For this review, take the finished solid that the model builds, in its own axes (mm). A direction names the side the tool comes from. Give positions to 0.01 mm unless a question says otherwise; leave off trailing zeros. Loops run counter-clockwise (first coordinate to the right, second up) from the corner with the lowest first, then second, coordinate; pieces in that order, holes last. Notation, with made-up numbers: (-23, 48.5) - (19, 48.5) arc R17 cw to (19, 62.5) - close; hole circle Ø11 at (17, -38.75). An arc over 180 degrees is marked (long way). Use CSV: the item, a comma, the result in double quotes. Start each with the question number.
1. Take a section at A-A on x = 22.5. Give the boundary of the cut face in (y, z).
2. For pin 1 (0.9 mm diameter, centred on x = 12, y = 1, fed in from -Z); pin 2 (1.4 mm diameter, centred on y = 0.5, z = -20, fed in from +X); pin 3 (2 mm diameter, centred on y = 1.5, z = -13, fed in from -X); pin 4 (0.5 mm diameter, centred on x = 31, y = -0.5, fed in from -Z), all flat-tipped, find the tip position at first contact; note any pin that passes through.
3. Wall thickness on line 1 (X direction, y = 0.7, z = -13); line 2 (Y direction, x = 11.5, z = -18.5); line 3 (Z direction, x = 6, y = 0.75): over which ranges is each line inside the solid? List them lowest first.
4. Take a section at B-B on z = -28. Give the boundary of the cut face in (x, y), plus the area to 3 significant figures.
5. Take a section at D-D on y = 1.1. Give the boundary of the cut face in (x, z) (1 decimal), plus the area to 3 significant figures.
6. Take a section at C-C on y = -0.7. Give the boundary of the cut face in (x, z).
7. Mouldability with a two-part tool opening along Z and no side actions: class faces 5 (the cylindrical face through (2.338, -1.526, -2.322)), 6 (the cylindrical face through (2.322, -1.526, -30.022)), 7 (the flat face through (15, 1, -1.613)), 8 (the flat face through (-1, -1, -23.038)) as pulls with the +Z half, pulls with the -Z half, needs draft (parallel to the pull), parting line crosses it, or undercut.
8. For faces 1 (the flat face through (0, -1, -27)), 2 (the flat face through (31, -1, -23.038)), 3 (the flat face through (30.048, -1, -5)), 4 (the flat face through (29.286, 1, -16)), list the 3-axis set-ups (+Z, -Z, +X, -X, +Y, -Y) from which the entire face can be reached by the end or side of a thin tool; tool diameter is ignored.
```python
from build123d import *

# Parameters (mm, degrees)
F1_DEPTH = 1.6764
F3_DEPTH = 0.3048
F5_DEPTH = 1.778


with BuildPart() as f1:
    # F0 (on Front) → F1 (new body)
    with BuildSketch(Plane.XZ):
        with BuildLine():
            Line((29.0322, 0), (1.016, 0))
            ThreePointArc((1.016, 0), (0.29758, -0.29758), (0, -1.016))
            Line((0, -1.016), (0, -8.3058))
            ThreePointArc((0, -8.3058), (-0.14879, -8.66501), (-0.508, -8.8138))
            Line((-0.508, -8.8138), (-1.524, -8.8138))
            ThreePointArc((-1.524, -8.8138), (-1.88321, -8.96259), (-2.032, -9.3218))
            Line((-2.032, -9.3218), (-2.032, -22.5298))
            ThreePointArc((-2.032, -22.5298), (-1.88321, -22.88901), (-1.524, -23.0378))
            Line((-1.524, -23.0378), (-0.508, -23.0378))
            ThreePointArc((-0.508, -23.0378), (-0.14879, -23.18659), (0, -23.5458))
            Line((0, -23.5458), (0, -31.3436))
            ThreePointArc((0, -31.3436), (0.29758, -32.06202), (1.016, -32.3596))
            Line((1.016, -32.3596), (29.0322, -32.3596))
            ThreePointArc((29.0322, -32.3596), (29.75062, -32.06202), (30.0482, -31.3436))
            Line((30.0482, -31.3436), (30.0482, -23.5458))
            ThreePointArc((30.0482, -23.5458), (30.19699, -23.18659), (30.5562, -23.0378))
            Line((30.5562, -23.0378), (31.5722, -23.0378))
            ThreePointArc((31.5722, -23.0378), (31.93141, -22.88901), (32.0802, -22.5298))
            Line((32.0802, -22.5298), (32.0802, -9.8298))
            ThreePointArc((32.0802, -9.8298), (31.93141, -9.47059), (31.5722, -9.3218))
            Line((31.5722, -9.3218), (30.5562, -9.3218))
            ThreePointArc((30.5562, -9.3218), (30.19699, -9.17301), (30.0482, -8.8138))
            Line((30.0482, -8.8138), (30.0482, -1.016))
            ThreePointArc((30.0482, -1.016), (29.75062, -0.29758), (29.0322, 0))
        make_face()
    extrude(amount=F1_DEPTH)

    # F2 (on face) → F3 (cut)
    with BuildSketch(Plane.XZ.offset(1.6764)):
        with BuildLine():
            Line((27.0002, -2.032), (3.048, -2.032))
            ThreePointArc((3.048, -2.032), (2.32958, -2.32958), (2.032, -3.048))
            Line((2.032, -3.048), (2.032, -29.3116))
            ThreePointArc((2.032, -29.3116), (2.32958, -30.03002), (3.048, -30.3276))
            Line((3.048, -30.3276), (27.0002, -30.3276))
            ThreePointArc((27.0002, -30.3276), (27.71862, -30.03002), (28.0162, -29.3116))
            Line((28.0162, -29.3116), (28.0162, -3.048))
            ThreePointArc((28.0162, -3.048), (27.71862, -2.32958), (27.0002, -2.032))
        make_face()
    extrude(amount=-F3_DEPTH, mode=Mode.SUBTRACT)

    # F4 (on face) → F5 (join)
    with BuildSketch(Plane(origin=(0, 0, 0), x_dir=(-1, 0, 0), z_dir=(0, 1, 0))):
        with BuildLine():
            Line((-2.3495, -1.6129), (-27.6987, -1.6129))
            ThreePointArc((-27.6987, -1.6129), (-28.821232, -2.077868), (-29.2862, -3.2004))
            Line((-29.2862, -3.2004), (-29.2862, -29.1592))
            ThreePointArc((-29.2862, -29.1592), (-28.821232, -30.281732), (-27.6987, -30.7467))
            Line((-27.6987, -30.7467), (-2.3495, -30.7467))
            ThreePointArc((-2.3495, -30.7467), (-1.226968, -30.281732), (-0.762, -29.1592))
            Line((-0.762, -29.1592), (-0.762, -3.2004))
            ThreePointArc((-0.762, -3.2004), (-1.226968, -2.077868), (-2.3495, -1.6129))
        make_face()
    extrude(amount=F5_DEPTH)


solid = f1.part
```
Check result:
1,outline,"(-1.68, -32.36) - (0, -32.36) - (0, -30.75) - (1.78, -30.75) - (1.78, -1.61) - (0, -1.61) - (0, 0) - (-1.68, 0) - (-1.68, -2.03) - (-1.37, -2.03) - (-1.37, -30.33) - (-1.68, -30.33) - close"
2,pin 1,"stops at z = -30.75"
2,pin 2,"stops at x = 32.08"
2,pin 3,"stops at x = 0.76"
2,pin 4,"stops at z = -23.04"
3,line 1,"x = 0.76 to 29.29"
3,line 2,"y = -1.37 to 1.78"
3,line 3,"z = -30.75 to -1.61"
4,outline,"(0, -1.68) - (2.03, -1.68) - (2.03, -1.37) - (28.02, -1.37) - (28.02, -1.68) - (30.05, -1.68) - (30.05, 0) - (29.29, 0) - (29.29, 1.78) - (0.76, 1.78) - (0.76, 0) - (0, 0) - close"
4,area,"93.2 mm²"
5,outline,"(0.8, -29.2) arc R1.6 ccw to (2.3, -30.7) - (27.7, -30.7) arc R1.6 ccw to (29.3, -29.2) - (29.3, -3.2) arc R1.6 ccw to (27.7, -1.6) - (2.3, -1.6) arc R1.6 ccw to (0.8, -3.2) - close"
5,area,"829 mm²"
6,outline,"(-2.03, -22.53) arc R0.51 ccw to (-1.52, -23.04) - (-0.51, -23.04) arc R0.51 cw to (0, -23.55) - (0, -31.34) arc R1.02 ccw to (1.02, -32.36) - (29.03, -32.36) arc R1.02 ccw to (30.05, -31.34) - (30.05, -23.55) arc R0.51 cw to (30.56, -23.04) - (31.57, -23.04) arc R0.51 ccw to (32.08, -22.53) - (32.08, -9.83) arc R0.51 ccw to (31.57, -9.32) - (30.56, -9.32) arc R0.51 cw to (30.05, -8.81) - (30.05, -1.02) arc R1.02 ccw to (29.03, 0) - (1.02, 0) arc R1.02 ccw to (0, -1.02) - (0, -8.31) arc R0.51 cw to (-0.51, -8.81) - (-1.52, -8.81) arc R0.51 ccw to (-2.03, -9.32) - close"
7,face 5,"undercut"
7,face 6,"undercut"
7,face 7,"pulls with the +Z half"
7,face 8,"pulls with the -Z half"
8,face 1,"-Z, -X, +Y, -Y"
8,face 2,"-Z, +X, +Y, -Y"
8,face 3,"+Z, +X, +Y, -Y"
8,face 4,"+Z, -Z, +X, +Y"
